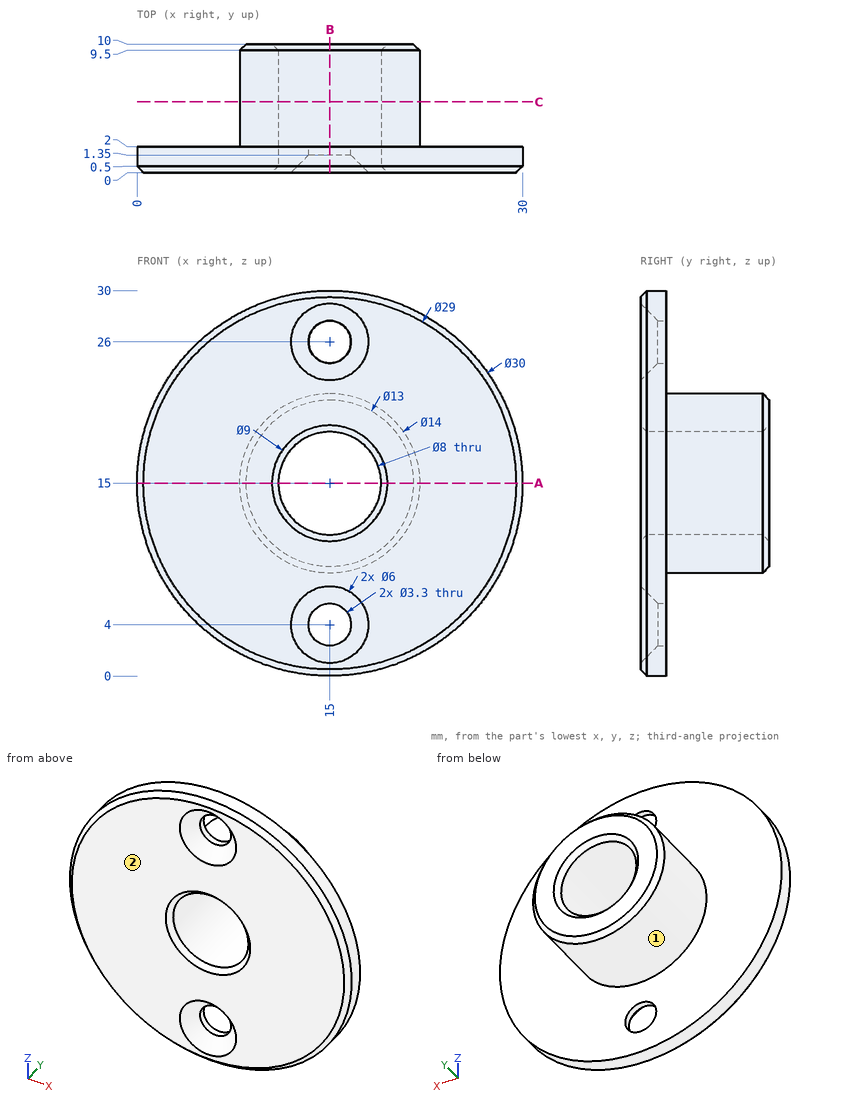
The drawing under review shows one solid part. Ordinate dimensions are in mm from its lowest x, y, z. A direction names the side the tool comes from. Round coordinates to 2 decimals unless told otherwise and drop trailing zeros. Order: outer loops, then holes, each group sorted by start corner. A loop starts at its lowest first (then second) coordinate and runs counter-clockwise, first axis right, second up. Notation, with made-up numbers: M -26.5,38.5 L 30.5,38.5 A22 ccw 30.5,72.5 Z; hole C -35,66.5 d7. An arc over 180 degrees is marked long. Answer as CSV lines item,"result". Start each with the question number.
1) Wall thickness on line 1 along X through (y, z) = (3.5, 15); line 2 along Y through (x, z) = (9, 10.75); line 3 along X through (y, z) = (1.55, 4): over which ranges is each line inside the solid? List them lowest first. Write a range as [from, to].
2) Tool access review of the marked faces 1 and 2: name each direction out of +Z, -Z, +X, -X, +Y, -Y from which nothing blocks a thin tool from reaching the whole face with its end or side.
3) Add section A-A (z = 15). Give the boundary of the cut face in (x, y), then the cut area to 3 significant figures.
4) For pin 1 Ø6 at (y, z) = (2, 6.5) entering from -X; pin 2 Ø10 at (x, z) = (11.5, 23.5) entering from +Y; pin 3 Ø5.5 at (x, z) = (15, 4) entering from +Y; pin 4 Ø4 at (y, z) = (6.5, 21.5) entering from +X, all flat-tipped, find the tip position at first contact; note any pin that passes through.
5) Add section B-B (x = 15). Give the number of separate pieces and of enclosed holes in the cut face, then the cut area to 3 significant figures.
6) Add section C-C (y = 5.5). Give the boundary of the cut face in (x, z).
Resolved:
1,line 1,"[8, 11], [19, 22]"
1,line 2,"[0, 2]"
1,line 3,"[4.8, 13.35], [16.65, 25.2]"
2,face 1,"+Y"
2,face 2,"+Z, -Z, +X, -X, -Y"
3,outline,"M 0,0.5 L 0.5,0 L 10.5,0 L 11,0.5 L 11,9.5 L 10.5,10 L 8.5,10 L 8,9.5 L 8,2 L 0,2 Z; M 19,0.5 L 19.5,0 L 29.5,0 L 30,0.5 L 30,2 L 22,2 L 22,9.5 L 21.5,10 L 19.5,10 L 19,9.5 Z"
3,area,"91.0 mm^2"
4,pin 1,"x = 1.04"
4,pin 2,"y = 10"
4,pin 3,"y = 2"
4,pin 4,"x = 20.36"
5,separate pieces,"4"
5,enclosed holes,"0"
5,area,"74.2 mm^2"
6,outline,"C 15,15 d14; hole C 15,15 d8"
